Autodesk Inventor part; units mm, degrees
ref_plane "YZ Plane" through (0, 0, 0) normal (1, 0, 0) x (0, 1, 0)
ref_plane "XZ Plane" through (0, 0, 0) normal (0, 1, 0) x (-1, 0, 0)
ref_plane "XY Plane" through (0, 0, 0) normal (0, 0, 1) x (1, 0, 0)
sketch "Эскиз1" plane through (0, 0, 0) normal (0, 0, 1) x (1, 0, 0)
  circle A0 centre (-4.8391, -17.7214) radius 1.5
  point P0 (0, 0)
extrude "Выдавливание1" add sketch "Эскиз1" against normal blind 30
sketch "Эскиз2" plane through (-4.8391, -17.7214, 0) normal (0, 0, 1) x (1, 0, 0)
  circle A0 centre (0, 0) radius 2.816
  point P0 (4.8391, 17.7214)
extrude "Выдавливание2" add sketch "Эскиз2" along normal blind 2
fillet "Сопряжение1" radius 1.7 1 edges at (-7.6551, -17.7214, 2)
sketch "Эскиз3" plane through (-4.8391, -17.7214, 2) normal (0, 0, 1) x (1, 0, 0)
  line L0 (-0.5, -1.9) -> (0.5, -1.9)
  line L1 (0.5, 1.9) -> (-0.5, 1.9)
  line L2 (1.9, -0.5) -> (1.9, 0.5)
  line L3 (-1.9, 0.5) -> (-1.9, -0.5)
  line L4 (-0.5, 1.9) -> (-0.5, 0.5)
  line L5 (-0.5, -0.5) -> (-0.5, -1.9)
  line L6 (1.9, 0.5) -> (0.5, 0.5)
  line L7 (-0.5, 0.5) -> (-1.9, 0.5)
  line L8 (0.5, -1.9) -> (0.5, -0.5)
  line L9 (0.5, 0.5) -> (0.5, 1.9)
  line L10 (-1.9, -0.5) -> (-0.5, -0.5)
  line L11 (0.5, -0.5) -> (1.9, -0.5)
  point P0 (4.8391, 17.7214)
  point P1 (0, 0)
extrude "Выдавливание3" cut sketch "Эскиз3" against normal blind 1.5
thread "Резьба1"
properties part number "Винт М3х30"
The listing builds one solid part. Answer for the finished solid, in the listing's coordinates (mm). A direction names the side the tool comes from. Coordinates: 2 decimals unless noted, no trailing zeros. Loops run counter-clockwise (first coordinate to the right, second up) from the corner with the lowest first, then second, coordinate; pieces in that order, holes last. Notation, with made-up numbers: (28.5, 55.25) - (46.5, 55.25) arc R14 ccw to (46.5, 78.25) - close; hole circle Ø10 at (32.25, 80). An arc over 180 degrees is marked (long way). Use a Markdown table: item, result. Add a question column.
1) The part is cut by section A-A, the plane z = -7. Give the vertices of the cut face in (x, y).
2) Find the intervals of material crossed by line 1 (Z direction, x = -6.25, y = -17.4); line 2 (Y direction, x = -4.8, z = -5); line 3 (Y direction, x = -3.5, z = -22), in increasing order.
3) For faces 4 (the cylindrical face through (-3.33, -20.1, 0.15)), 5 (the flat face through (-5.339, -19, 1)), determine the directions among +Z, -Z, +X, -X, +Y, -Y from which every point of the face is accessible in a straight line to the end or side of a thin tool.
4) The mould has two halves that part along X. Classify faces 1 (the flat face through (-3.6, -18.9, 0)), 2 (the cylindrical face through (-4.03, -16.46, -14.79)), 3 (the flat face through (-6, -18.221, 1)): released by +X, released by -X, zero draft, split by the parting line, or undercut.
5) Given pin 1 (0.8 mm diameter, centred on x = -5, z = 1.5, fed in from +Y); pin 2 (1.1 mm diameter, centred on y = -17.5, z = 1, fed in from +X); pin 3 (1.9 mm diameter, centred on x = -4.5, y = -17.5, fed in from +Z); pin 4 (2 mm diameter, centred on y = -20, z = -13, fed in from -X), each flat-ended and moving along its own axis, determine where each tip first touches the part or whether it passes through.
Here are the results:
| question | item | result |
|---|---|---|
| 1 | outline | circle Ø3 at (-4.84, -17.72) |
| 2 | line 1 | z = -30 to 0.5 |
| 2 | line 2 | y = -19.22 to -16.22 |
| 2 | line 3 | y = -18.4 to -17.05 |
| 3 | face 4 | +Z, -Z |
| 3 | face 5 | +Z |
| 4 | face 1 | zero draft |
| 4 | face 2 | split by the parting line |
| 4 | face 3 | undercut |
| 5 | pin 1 | stops at y = -15.11 |
| 5 | pin 2 | stops at x = -2.03 |
| 5 | pin 3 | stops at z = 2 |
| 5 | pin 4 | stops at x = -5.62 |
